The figure shows three views and two pictorial views of one solid part (mm, origin at its lowest corner). Answer the questions. A direction names the side the tool comes from. Round coordinates to 2 decimals unless told otherwise and drop trailing zeros. Order: outer loops, then holes, each group sorted by start corner. A loop starts at its lowest first (then second) coordinate and runs counter-clockwise, first axis right, second up. Notation, with made-up numbers: (-11.5, 34.25) -> (14.5, 34.25) arc R17 ccw to (14.5, 45.25) -> close; hole circle Ø4 at (25, 54.5). An arc over 180 degrees is marked (long way). One line per item, written item: value. Start each with the question number.
1. Consider line 1 (Z direction, x = 21.2, y = 5); line 2 (Y direction, x = 20.05, z = 5); line 3 (X direction, y = 9, z = 12). Determine where each line is inside the solid, lowest interval first.
2. Section D-D (y = 11) is taken. Give the vertices of the cut face in (x, z).
3. The mould has two halves that part along X. Classify the marked faces 1, 2, 3 and 4: released by +X, released by -X, zero draft, split by the parting line, or undercut.
4. For the marked faces 5, 6, 7 and 8, determine the directions among +Z, -Z, +X, -X, +Y, -Y from which every point of the face is accessible in a straight line to the end or side of a thin tool.
5. Section B-B (x = 8) is taken. Give the vertices of the cut face in (y, z).
6. Flat-ended cylindrical pins translate along their axes: pin 1 Ø2.5 at (x, y) = (9, 9) entering from -Z; pin 2 Ø8 at (x, z) = (13.5, 6.5) entering from +Y; pin 3 Ø5 at (y, z) = (5, 5) entering from -X; pin 4 Ø2.5 at (x, y) = (8.5, 9) entering from +Z. Find the tip coordinate at first contact, or state that the pin passes through.
7. Section A-A (y = 9) is taken. Give the vertices of the cut face in (x, z), then the cut area to 3 significant figures.
8. Section C-C (z = 5) is taken. Give the vertices of the cut face in (x, y), then the cut area to 3 significant figures.
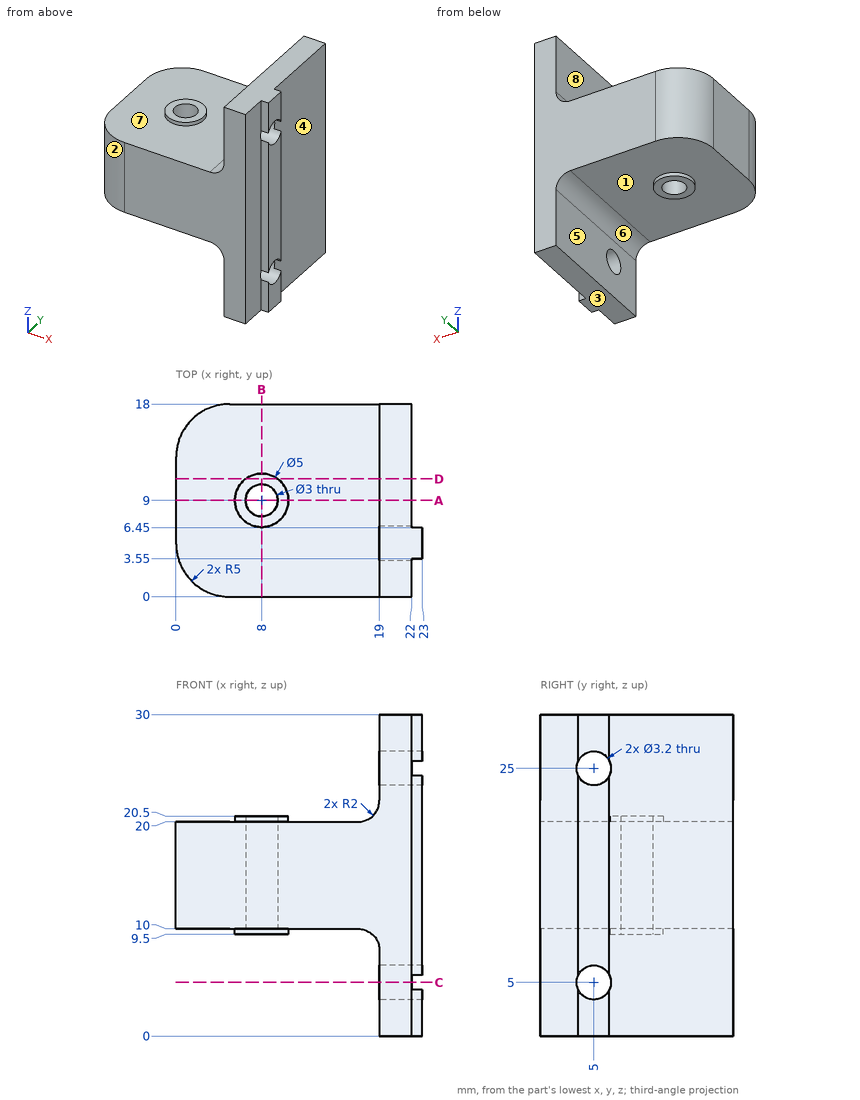
Answer:
1. line 1: 0 to 3.4, 6.6 to 23.4, 26.6 to 30
1. line 2: 0 to 3.4, 6.6 to 18
1. line 3: 0 to 6.5, 9.5 to 22
2. outline: (0, 10) -> (6.5, 10) -> (6.5, 9.5) -> (9.5, 9.5) -> (9.5, 10) -> (17, 10) arc R2 cw to (19, 8) -> (19, 0) -> (22, 0) -> (22, 30) -> (19, 30) -> (19, 22) arc R2 cw to (17, 20) -> (9.5, 20) -> (9.5, 20.5) -> (6.5, 20.5) -> (6.5, 20) -> (0, 20) -> close
3. face 1: undercut
3. face 2: released by -X
3. face 3: zero draft
3. face 4: released by +X
4. face 5: -Z, -X, +Y, -Y
4. face 6: -Z, +Y, -Y
4. face 7: +Z
4. face 8: +Z, -X, +Y, -Y
5. outline: (0, 10) -> (6.5, 10) -> (6.5, 9.5) -> (7.5, 9.5) -> (7.5, 20.5) -> (6.5, 20.5) -> (6.5, 20) -> (0, 20) -> close; (10.5, 9.5) -> (11.5, 9.5) -> (11.5, 10) -> (18, 10) -> (18, 20) -> (11.5, 20) -> (11.5, 20.5) -> (10.5, 20.5) -> close
6. pin 1: z = 9.5
6. pin 2: y = 18
6. pin 3: x = 19
6. pin 4: z = 20.5
7. outline: (0, 10) -> (5.5, 10) -> (5.5, 9.5) -> (6.5, 9.5) -> (6.5, 20.5) -> (5.5, 20.5) -> (5.5, 20) -> (0, 20) -> close; (9.5, 9.5) -> (10.5, 9.5) -> (10.5, 10) -> (17, 10) arc R2 cw to (19, 8) -> (19, 0) -> (22, 0) -> (22, 30) -> (19, 30) -> (19, 22) arc R2 cw to (17, 20) -> (10.5, 20) -> (10.5, 20.5) -> (9.5, 20.5) -> close
7. area: 254 mm^2
8. outline: (19, 0) -> (22, 0) -> (22, 3.4) -> (19, 3.4) -> close; (19, 6.6) -> (22, 6.6) -> (22, 18) -> (19, 18) -> close
8. area: 44.4 mm^2
